Geometry check sheet. Reference: the model listing, model coordinates, mm. A direction names the side the tool comes from. Coordinates: 2 decimals unless noted, no trailing zeros. Write each loop counter-clockwise with the first axis right and the second up, starting at its lowest first coordinate (ties: lowest second). Pieces come first, ordered by that corner, then holes.
from build123d import *

# Parameters (mm, degrees)
SKIZZE1_W                                           = 135.069444444
SKIZZE1_H                                           = 100
AUFSATZ_LINEAR_AUSTRAGEN1_DEPTH                     = 40
SCHNITT_LINEAR_AUSTRAGEN1_DEPTH                     = 150.47827542
SCHNITT_LINEAR_AUSTRAGEN2_DEPTH                     = 128.125680748
STIRNSENKUNG_F_R_M8_SENKSCHRAUBE_KOPF_B_D           = 9
STIRNSENKUNG_F_R_M8_SENKSCHRAUBE_KOPF_B_CBORE_D     = 15
STIRNSENKUNG_F_R_M8_SENKSCHRAUBE_KOPF_B_CBORE_DEPTH = 35


with BuildPart() as part:
    # Skizze1 → Aufsatz-Linear austragen1 (new body)
    with BuildSketch(Plane.XY):
        Rectangle(SKIZZE1_W, SKIZZE1_H)
    extrude(amount=AUFSATZ_LINEAR_AUSTRAGEN1_DEPTH)

    # Skizze2 → Schnitt-Linear austragen1 (cut, through all)
    with BuildSketch(Plane(origin=(67.534722222, 0, 0), x_dir=(0, 0, -1), z_dir=(1, 0, 0))):
        with BuildLine():
            Line((-5, 50), (42.421873459, 50))
            Line((42.421873459, 50), (-56.728012939, 80.829845409))
            Line((-56.728012939, 80.829845409), (-40, -11.655385644))
            Line((-40, -11.655385644), (-40, 15))
            ThreePointArc((-40, 15), (-29.748737342, 39.748737342), (-5, 50))
        make_face()
    schnitt_linear_austragen1 = extrude(amount=-SCHNITT_LINEAR_AUSTRAGEN1_DEPTH, mode=Mode.SUBTRACT)

    # Spiegeln1: Schnitt-Linear austragen1 across plane
    add(schnitt_linear_austragen1.mirror(Plane.ZX), mode=Mode.SUBTRACT)

    # Skizze5 → Schnitt-Linear austragen2 (cut, through all)
    with BuildSketch(Plane(origin=(0, 50, 0), x_dir=(1, 0, 0), z_dir=(0, 1, 0))):
        with BuildLine():
            Line((-67.534722222, -5), (-67.534722222, -19.872389704))
            Line((-67.534722222, -19.872389704), (-98.364567631, -61.728012939))
            Line((-98.364567631, -61.728012939), (-5.879336578, -40))
            Line((-5.879336578, -40), (-32.534722222, -40))
            ThreePointArc((-32.534722222, -40), (-57.283459564, -29.748737342), (-67.534722222, -5))
        make_face()
    schnitt_linear_austragen2 = extrude(amount=-SCHNITT_LINEAR_AUSTRAGEN2_DEPTH, mode=Mode.SUBTRACT)

    # Spiegeln2: Schnitt-Linear austragen2 across plane
    add(schnitt_linear_austragen2.mirror(Plane(origin=(0, 0, 0), x_dir=(0, 0, 1), z_dir=(1, 0, 0))), mode=Mode.SUBTRACT)

    # Stirnsenkung für M8 Senkschraube (Kopf Button)3 (through all)
    with Locations(Plane.XY.offset(40)):
        with Locations((0, -30)):
            stirnsenkung_f_r_m8_senkschraube_kopf_b = CounterBoreHole(STIRNSENKUNG_F_R_M8_SENKSCHRAUBE_KOPF_B_D / 2, STIRNSENKUNG_F_R_M8_SENKSCHRAUBE_KOPF_B_CBORE_D / 2, STIRNSENKUNG_F_R_M8_SENKSCHRAUBE_KOPF_B_CBORE_DEPTH)

    # Spiegeln5: Stirnsenkung für M8 Senkschraube (Kopf Button)3 across plane
    add(stirnsenkung_f_r_m8_senkschraube_kopf_b.mirror(Plane.ZX), mode=Mode.SUBTRACT)


solid = part.part
1. Sectioned sample at A-A, the plane y = -30. Record the boundary of the cut face in (x, z), and give its area (3 significant figures).
Computed values:
outline: (-67.53, 0) - (-4.5, 0) - (-4.5, 5) - (-7.5, 5) - (-7.5, 36.62) - (-47.53, 36.62) arc R35 ccw to (-67.53, 5) - close; (4.5, 0) - (67.53, 0) - (67.53, 5) arc R35 ccw to (47.53, 36.62) - (7.5, 36.62) - (7.5, 5) - (4.5, 5) - close
area: 4,070 mm2
2. Gauge pin test, flat ends, axial feed: pin 1 Ø6 at (x, z) = (29.5, 15.5) entering from -Y; pin 2 Ø2 at (x, z) = (-34.5, 10.5) entering from +Y; pin 3 Ø10 at (y, z) = (-16, 33) entering from -X. Record the tip position at first contact, or that the pin passes through.
Computed values:
pin 1: stops at y = -49.19
pin 2: stops at y = 49.71
pin 3: stops at x = -58.92
3. Sectioned sample at C-C, the plane z = 30. Record the boundary of the cut face in (x, y), and give its area (3 significant figures).
Computed values:
outline: (-57.03, -39.49) - (57.03, -39.49) - (57.03, 39.49) - (-57.03, 39.49) - close; hole circle Ø15 at (0, -30); hole circle Ø15 at (0, 30)
area: 8,660 mm2
4. Draft check along X on faces 3 (the flat face through (-67.535, -1, 2)), 4 (the flat face through (5, 30, 5)), 5 (the flat face through (0, 0, 40)). Enter one of: released by +X, released by -X, zero draft, split by the parting line, or undercut.
Computed values:
face 3: released by -X
face 4: undercut
face 5: zero draft
5. Thickness scan on line 1 along Y through (x, z) = (0, 22); line 2 along Y through (x, z) = (0, 30.5); line 3 along X through (y, z) = (13, 6). Record the ranges inside material, lowest first.
Computed values:
line 1: y = -45.59 to -37.5, -22.5 to 22.5, 37.5 to 45.59
line 2: y = -38.97 to -37.5, -22.5 to 22.5, 37.5 to 38.97
line 3: x = -67.52 to 67.52
6. Sectioned sample at D-D, the plane x = 14. Record the boundary of the cut face in (y, z), and give its area (3 significant figures).
Computed values:
outline: (-50, 0) - (50, 0) - (50, 5) arc R35 ccw to (15, 40) - (-15, 40) arc R35 ccw to (-50, 5) - close
area: 3,470 mm2
7. Access from +Z, -Z, +X, -X, +Y, -Y to the whole of each face (thin tool, end or side, straight path). Record for faces 1 (the flat face through (67.535, -1, 2)), 2 (the cylindrical face through (-0.976, 22.564, 22.333)).
Computed values:
face 1: +Z, -Z, +X, +Y, -Y
face 2: +Z
8. Sectioned sample at B-B, the plane x = 0. Record the boundary of the cut face in (y, z), and give its area (3 significant figures).
Computed values:
outline: (-50, 0) - (-34.5, 0) - (-34.5, 5) - (-37.5, 5) - (-37.5, 31.81) arc R35 ccw to (-50, 5) - close; (-25.5, 0) - (25.5, 0) - (25.5, 5) - (22.5, 5) - (22.5, 39.19) arc R35 ccw to (15, 40) - (-15, 40) arc R35 ccw to (-22.5, 39.19) - (-22.5, 5) - (-25.5, 5) - close; (34.5, 0) - (50, 0) - (50, 5) arc R35 ccw to (37.5, 31.81) - (37.5, 5) - (34.5, 5) - close
area: 2,450 mm2
